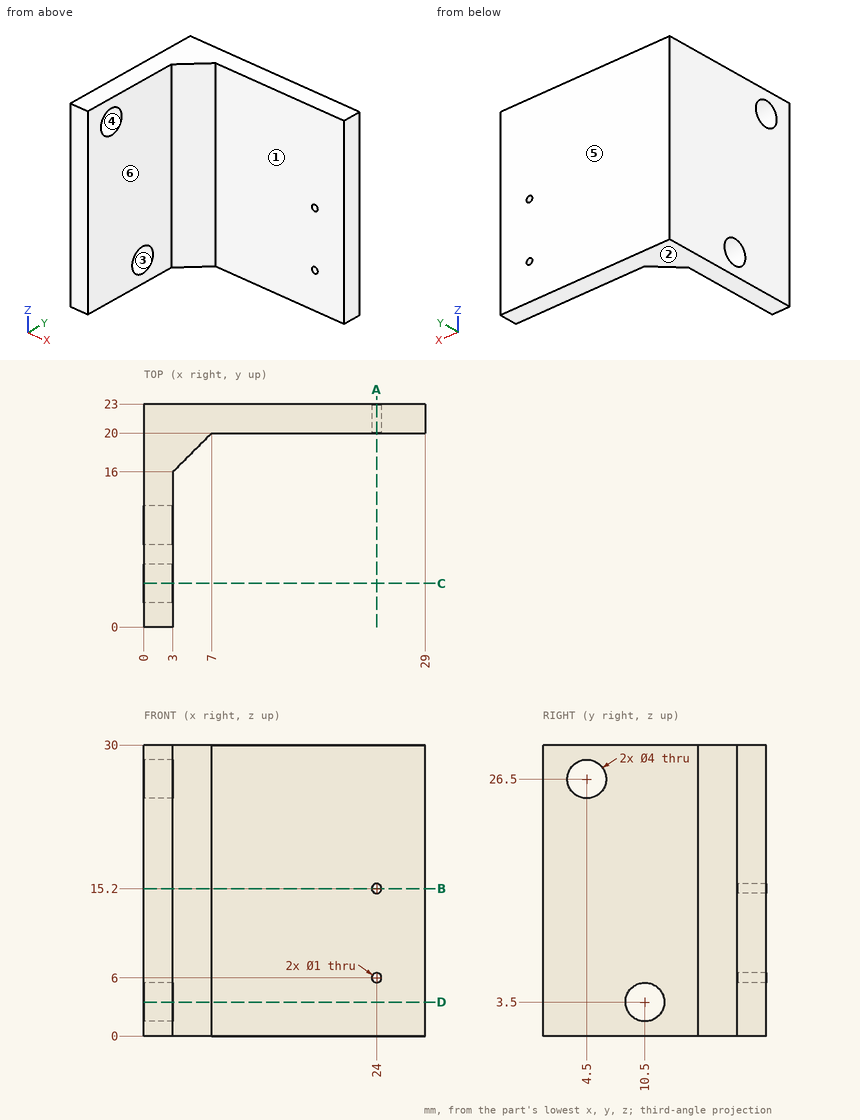
For this review, use the dimensioned drawing (mm, ordinates from the lowest corner) and the shaded views. A direction names the side the tool comes from. Round coordinates to 2 decimals unless told otherwise and drop trailing zeros. Write each loop counter-clockwise with the first axis right and the second up, starting at its lowest first coordinate (ties: lowest second). Pieces come first, ordered by that corner, then holes. Notation, with made-up numbers: M 4.25,18.5 L 14.25,18.5 A20 cw 14.25,56.5 Z; hole C -25.5,79 d6. An arc over 180 degrees is marked long. Write item = value, one per line. Start each with the question number.
(1) We need section D-D (z = 3.5). Give the boundary of the cut face in (x, y), then the cut area to 3 significant figures.
(2) We need section C-C (y = 4.5). Give the boundary of the cut face in (x, z), then the cut area to 3 significant figures.
(3) The part is to be moulded in two halves that separate along Y. For the marked faces 3, 4, 5 and 6, say which applies: +Y half, -Y half, draft (parallel to the pull), parting line (faces both ways), or undercut.
(4) Clearance check with flat-ended pins moving along their axes: pin 1 Ø6 at (y, z) = (2.5, 11.5) entering from +X; pin 2 Ø4.5 at (y, z) = (10.5, 3.5) entering from -X. State where each tip first meets the part, or that it passes through.
(5) We need section B-B (z = 15.2). Give the boundary of the cut face in (x, y), then the cut area to 3 significant figures.
(6) For line 1 along Z through (x, y) = (24, 22); line 2 along X through (y, z) = (22.3, 15.2); line 3 along Y through (x, z) = (1.35, 26.5), list the stretches that pass through material, from the lowest coordinate up.
(7) We need section A-A (x = 24). Give the boundary of the cut face in (y, z).
(8) For the marked faces 1 and 2, list the 3-axis set-ups (+Z, -Z, +X, -X, +Y, -Y) from which the entire face can be reached by the end or side of a thin tool; tool diameter is ignored.
Results found:
q1.outline = M 0,0 L 3,0 L 3,8.5 L 0,8.5 Z; M 0,12.5 L 3,12.5 L 3,16 L 7,20 L 29,20 L 29,23 L 0,23 Z
q1.area = 143 mm²
q2.outline = M 0,0 L 3,0 L 3,24.5 L 0,24.5 Z; M 0,28.5 L 3,28.5 L 3,30 L 0,30 Z
q2.area = 78.0 mm²
q3.face_3 = undercut
q3.face_4 = undercut
q3.face_5 = +Y half
q3.face_6 = draft
q4.pin_1 = 3
q4.pin_2 = 0
q5.outline = M 0,0 L 3,0 L 3,16 L 7,20 L 23.5,20 L 23.5,23 L 0,23 Z; M 24.5,20 L 29,20 L 29,23 L 24.5,23 Z
q5.area = 152 mm²
q6.line_1 = 0 to 5.5, 6.5 to 14.7, 15.7 to 30
q6.line_2 = 0 to 23.5, 24.5 to 29
q6.line_3 = 0 to 2.5, 6.5 to 23
q7.outline = M 20,0 L 23,0 L 23,5.5 L 20,5.5 Z; M 20,6.5 L 23,6.5 L 23,14.7 L 20,14.7 Z; M 20,15.7 L 23,15.7 L 23,30 L 20,30 Z
q8.face_1 = +Z, -Z, +X, -Y
q8.face_2 = -Z, +X, -X, +Y, -Y
